```python
from build123d import *

# Parameters (mm, degrees)
F0_W     = 101.6
F0_H     = 38.1
F2_DEPTH = 63.5
F1_W     = 34.0687744319
F1_H     = 0.7092284867
F1_H_2   = 37.4890945023
F3_DEPTH = 37.592
F5_DEPTH = 12.192
F7_DEPTH = 50.8


with BuildPart() as f2:
    # F0 (on Top) → F2 (new body)
    with BuildSketch(Plane.XY):
        with Locations((2.7100164443, -7.8571270815)):
            Rectangle(F0_W, F0_H)
    extrude(amount=F2_DEPTH)

    # F1 (on face) → F3 (cut)
    with BuildSketch(Plane.XY):
        with Locations((2.0647738129, -27.2617413248)):
            Rectangle(F1_W, F1_H)
        with Locations((2.0647738129, -8.1625798303)):
            Rectangle(F1_W, F1_H_2)
    extrude(amount=F3_DEPTH, mode=Mode.SUBTRACT)

    # F4 (on face) → F5 (cut)
    with BuildSketch(Plane(origin=(0, 0, 0), x_dir=(1, 0, 0), z_dir=(0, 0, -1))):
        Polygon((-48.0899835557, -11.1928729185), (-14.9696134031, -11.1928729185), (-14.9696134031, -10.5819674209), (-14.9696134031, 26.9071270815), (-48.0899835557, 26.9071270815), align=None)
    extrude(amount=-F5_DEPTH, mode=Mode.SUBTRACT)

    # F6 (on face) → F7 (cut)
    with BuildSketch(Plane.XZ.offset(26.9071270815)):
        Polygon((-48.0899835557, 12.192), (-31.5297984794, 12.192), (-48.0899835557, 37.846), align=None)
    extrude(amount=-F7_DEPTH, mode=Mode.SUBTRACT)


solid = f2.part
```
Geometry check sheet. Reference: the model listing, model coordinates, mm. A direction names the side the tool comes from. Coordinates: 2 decimals unless noted, no trailing zeros. Loops run counter-clockwise (first coordinate to the right, second up) from the corner with the lowest first, then second, coordinate; pieces in that order, holes last. Notation, with made-up numbers: (67.25, -33) - (83.25, -33) arc R24 cw to (83.25, -17) - close; hole circle Ø2 at (-17.75, 72). An arc over 180 degrees is marked (long way). One line per item, written item: value. Start each with the question number.
(1) Cross-section at D-D on z = 33.5. Enter the section's corners in (x, y).
(2) Cross-section at A-A on z = 25. Enter the section's corners in (x, y), plus the area to 3 significant figures.
(3) Cross-section at C-C on x = -25. Enter the section's corners in (y, z), plus the area to 3 significant figures.
(4) Depth check by flat-ended pin: P1, Ø10, axis at x = 3.5, y = -2.5, coming from the -Z side; P2, Ø1, axis at y = -8, z = 15, coming from the -X side; P3, Ø11, axis at y = 0.5, z = 24.5, coming from the -X side. Enter the tip coordinate at first touch or a pass-through.
(5) Cross-section at B-B on y = -8.5. Enter the section's corners in (x, z), plus the area to 3 significant figures.
(6) Mould release check, pull along X, two halves, no side actions. Record for faces 4 (the flat face through (53.51, -8, 31)), 5 (the flat face through (2, 11.193, 31)), 6 (the flat face through (19.099, -8, 19)): released by +X, released by -X, zero draft, split by the parting line, or undercut.
(7) Material ranges on line 1 (Y direction, x = 18, z = 11); line 2 (Z direction, x = 14, y = -1.5); line 3 (X direction, y = 5.5, z = 24), recorded low to high. Write a range as [from, to].
(8) Tool access check on faces 1 (the flat face through (2, -8, 37.592)), 2 (the flat face through (-23, -8, 12.192)), 3 (the flat face through (2, -8, 63.5)). Record the directions out of +Z, -Z, +X, -X, +Y, -Y that give a thin tool (end or side, any length) a straight path to the whole face; none if there is none.
Results below:
1. outline: (-45.28, -26.91) - (-14.97, -26.91) - (-14.97, 10.58) - (19.1, 10.58) - (19.1, -26.91) - (53.51, -26.91) - (53.51, 11.19) - (-45.28, 11.19) - close
2. outline: (-39.8, -26.91) - (-14.97, -26.91) - (-14.97, 10.58) - (19.1, 10.58) - (19.1, -26.91) - (53.51, -26.91) - (53.51, 11.19) - (-39.8, 11.19) - close
2. area: 2,280 mm2
3. outline: (-26.91, 12.19) - (11.19, 12.19) - (11.19, 63.5) - (-26.91, 63.5) - close
3. area: 1,950 mm2
4. P1: stops at z = 37.59
4. P2: stops at x = -33.67
4. P3: stops at x = -43.03
5. outline: (-48.09, 37.85) - (-31.53, 12.19) - (-14.97, 12.19) - (-14.97, 37.59) - (19.1, 37.59) - (19.1, 0) - (53.51, 0) - (53.51, 63.5) - (-48.09, 63.5) - close
5. area: 4,550 mm2
6. face 4: released by +X
6. face 5: zero draft
6. face 6: undercut
7. line 1: y = [10.58, 11.19]
7. line 2: z = [37.59, 63.5]
7. line 3: x = [-39.15, -14.97], [19.1, 53.51]
8. face 1: -Z, -Y
8. face 2: -Z, -X, +Y, -Y
8. face 3: +Z, +X, -X, +Y, -Y
